Geometry: final body of the model. Coordinates: model frame, mm. Give positions to 0.01 mm unless a question says otherwise; leave off trailing zeros. Order: outer loops, then holes, each group sorted by start corner. A loop starts at its lowest first (then second) coordinate and runs counter-clockwise, first axis right, second up. Notation, with made-up numbers: (45.5, 87) -> (93.5, 87) arc R30 cw to (93.5, 110) -> close; hole circle Ø6 at (20, 20). An arc over 180 degrees is marked (long way). Answer in a Markdown table with one row per item. Add a question column.
Q1. Cut plane A-A on z = 24. Return the cut outline in (x, y), and give its area (3 significant figures).
Q2. Cut plane B-B on y = 2. Count the separate pieces of the cut face and the enclosed holes in it, and give its area (3 significant figures).
Q3. Line query: line 1 along X through (y, z) = (3.75, 27); line 2 along X through (y, z) = (1.3, 17.5); line 3 along Z through (x, y) = (17.5, 4.2). Output: solid intervals per line, ascending. Write a range as from..to.
Q4. Contact query for a flat-ended pin moving along its axis: P1, Ø3, axis at x = 25, z = 9, coming from the +Y side. Output: stop coordinate, or through.
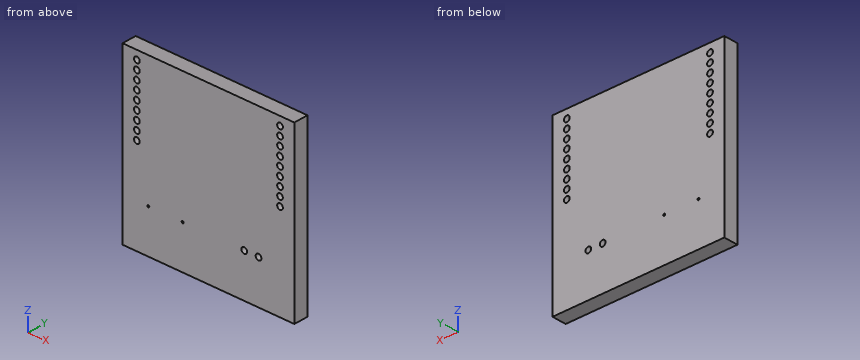
Autodesk Inventor part; units mm, degrees
ref_plane "YZ Plane" through (0, 0, 0) normal (1, 0, 0) x (0, 1, 0)
ref_plane "XZ Plane" through (0, 0, 0) normal (0, 1, 0) x (-1, 0, 0)
ref_plane "XY Plane" through (0, 0, 0) normal (0, 0, 1) x (1, 0, 0)
sketch "Эскиз1" plane through (0, 0, 0) normal (0, 1, 0) x (-1, 0, 0)
  line L0 (0, 30) -> (30, 30)
  line L1 (30, 30) -> (30, -30)
  line L2 (30, -30) -> (-20, -30)
  line L3 (-20, 30) -> (0, 30)
  line L4 (-30, 0) -> (-30, -30)
  line L5 (-30, -30) -> (-30, 30)
  line L6 (-20, 30) -> (-30, 30)
  line L7 (-30, -30) -> (-20, -30)
  point P0 (0, 0)
extrude "Выдавливание1" add sketch "Эскиз1" along normal blind 5
sketch "Эскиз2" plane through (0, 5, 0) normal (0, 1, 0) x (1, 0, 0)
  line L0 (-30, 30) -> (-30, -30)
  line L1 (-30, 0) -> (30, 0)
  line L2 (30, -30) -> (30, 30)
  line L3 (0, 0) -> (0, 30)
  line L4 (30, 30) -> (-30, 30)
  line L5 (0, 15) -> (30, 15)
  line L6 (15, 0) -> (15, 30)
  line L7 (15, 15) -> (12.5, 15)
  line L8 (12.5, 15) -> (17.5, 15)
  dimension "d46" = 2.5
  dimension "d47" = 5
sketch "Эскиз3" plane through (0, 5, 0) normal (0, 1, 0) x (1, 0, 0)
  line L0 (30, -30) -> (30, 30)
  line L1 (-30, -30) -> (30, -30)
  line L2 (25, 0) -> (25, -3)
  line L3 (25, -30) -> (25, -27)
  line L4 (-25, -27) -> (-25, -3)
  line L5 (-25, -27) -> (-25, -24)
  line L6 (-25, -24) -> (-25, -21)
  line L7 (-25, -21) -> (-25, -18)
  line L8 (-25, -18) -> (-25, -15)
  line L9 (-25, -15) -> (-25, -12)
  line L10 (-25, -12) -> (-25, -9)
  line L11 (-25, -9) -> (-25, -6)
  line L12 (25, -27) -> (25, -3)
  line L13 (25, -27) -> (25, -24)
  line L14 (25, -24) -> (25, -21)
  line L15 (25, -21) -> (25, -18)
  line L16 (25, -18) -> (25, -15)
  line L17 (25, -15) -> (25, -12)
  line L18 (25, -12) -> (25, -9)
  line L19 (25, -9) -> (25, -6)
  point P0 (0, 0)
  dimension "d19" = 3
  dimension "d20" = 3
  dimension "d21" = 3
  dimension "d22" = 3
  dimension "d23" = 3
  dimension "d24" = 3
  dimension "d25" = 3
  dimension "d26" = 3
  dimension "d27" = 3
  dimension "d28" = 3
hole "Отверстие1" at (-25, 5, 27) at (-25, 5, 24) at (-25, 5, 21) at (-25, 5, 18) at (-25, 5, 15) at (-25, 5, 12) at (-25, 5, 9) at (-25, 5, 6) at (-25, 5, 3) at (25, 5, 27) at (25, 5, 24) at (25, 5, 21) at (25, 5, 18) at (25, 5, 15) at (25, 5, 12) at (25, 5, 9) at (25, 5, 6) at (25, 5, 3) direction (0, -1, 0) diameter 2 end through all
sketch "Эскиз4" plane through (0, 5, 0) normal (0, 1, 0) x (1, 0, 0)
  line L0 (-30, 30) -> (-30, -30)
  line L1 (-30, 0) -> (-30, 15)
  line L2 (-30, 15) -> (0, 15)
  line L3 (-30, 15) -> (-21, 15)
  line L4 (0, 15) -> (-9, 15)
  point P0 (0, 0)
  dimension "d36" = 15
  dimension "d37" = 9
  dimension "d38" = 9
hole "Отверстие2" at (-21, 5, -15) at (-9, 5, -15) direction (0, -1, 0) diameter 0.7 end through all
hole "Отверстие3" at (12.5, 5, -15) at (17.5, 5, -15) direction (0, -1, 0) diameter 2 end through all
ref_plane "РабПлоскость1" through (30, 5, -30) normal (0, -0.7071, -0.7071) x (-1, 0, 0)
Completed:
| question | item | result |
|---|---|---|
| 1 | outline | (-30, 0) -> (-26, 0) -> (-26, 5) -> (-30, 5) -> close; (-24, 0) -> (24, 0) -> (24, 5) -> (-24, 5) -> close; (26, 0) -> (30, 0) -> (30, 5) -> (26, 5) -> close |
| 1 | area | 280 mm² |
| 2 | separate pieces | 1 |
| 2 | enclosed holes | 22 |
| 2 | area | 3,540 mm² |
| 3 | line 1 | x = -30..-26, -24..24, 26..30 |
| 3 | line 2 | x = -30..-25.87, -24.13..24.13, 25.87..30 |
| 3 | line 3 | z = -30..-16, -14..30 |
| 4 | P1 | stops at y = 5 |
